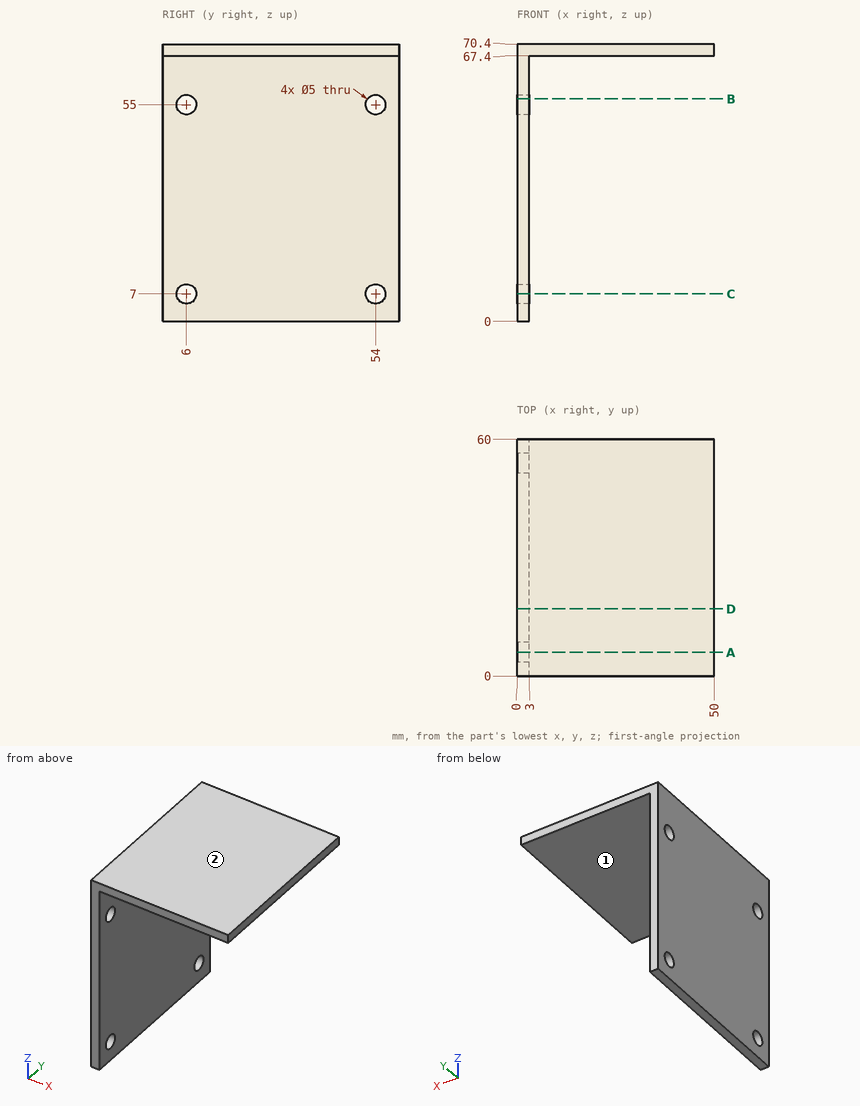
Job drawing, mm, ordinate dimensions from the low corner. One solid piece. A direction names the side the tool comes from. Round coordinates to 2 decimals unless told otherwise and drop trailing zeros. Write each loop counter-clockwise with the first axis right and the second up, starting at its lowest first coordinate (ties: lowest second). Pieces come first, ordered by that corner, then holes. Notation, with made-up numbers: (-21.75, 63.25) -> (-3.75, 63.25) arc R16 ccw to (-3.75, 88.25) -> close; hole circle Ø3 at (2, -22). An arc over 180 degrees is marked (long way). Answer as a JSON object with one key per item and string values.
(1) Which spindle directions (+Z, -Z, +X, -X, +Y, -Y) get a long thin tool onto all of the face, cutting with end or side? Do the marked faces 1 and 2. Say none if no direction does.
Reported:
{"face 1": "-Z, +X, +Y, -Y", "face 2": "+Z, +X, -X, +Y, -Y"}
(2) Band-saw the part on D-D, the plane y = 17. List the corners of the cut face in (x, z), then the cut area to 3 significant figures.
Reported:
{"outline": "(0, 0) -> (3, 0) -> (3, 67.4) -> (50, 67.4) -> (50, 70.4) -> (0, 70.4) -> close", "area": "352 mm^2"}
(3) Probe probe 1 along Y at (x, z) = (1.65, 7); probe 2 along X at (y, z) = (54.5, 47); probe 3 along Z at (x, y) = (46, 7). List the from-to ranges inside material, lowest first. Write a range as [from, to].
Reported:
{"probe 1": "y = [0, 3.5], [8.5, 51.5], [56.5, 60]", "probe 2": "x = [0, 3]", "probe 3": "z = [67.4, 70.4]"}
(4) Band-saw the part on C-C, the plane z = 7. List the corners of the cut face in (x, y).
Reported:
{"outline": "(0, 0) -> (3, 0) -> (3, 3.5) -> (0, 3.5) -> close; (0, 8.5) -> (3, 8.5) -> (3, 51.5) -> (0, 51.5) -> close; (0, 56.5) -> (3, 56.5) -> (3, 60) -> (0, 60) -> close"}
(5) Pin check, flat tips, straight feed: P1, Ø14, axis at x = 20.5, y = 32, coming from the -Z side; P2, Ø6.5, axis at y = 54, z = 55, coming from the +X side. Stop position of each tip, or through.
Reported:
{"P1": "stops at z = 67.4", "P2": "stops at x = 3"}
(6) Band-saw the part on B-B, the plane z = 56.5. List the corners of the cut face in (x, y).
Reported:
{"outline": "(0, 0) -> (3, 0) -> (3, 4) -> (0, 4) -> close; (0, 8) -> (3, 8) -> (3, 52) -> (0, 52) -> close; (0, 56) -> (3, 56) -> (3, 60) -> (0, 60) -> close"}
(7) Band-saw the part on A-A, the plane y = 6. List the corners of the cut face in (x, z).
Reported:
{"outline": "(0, 0) -> (3, 0) -> (3, 4.5) -> (0, 4.5) -> close; (0, 9.5) -> (3, 9.5) -> (3, 52.5) -> (0, 52.5) -> close; (0, 57.5) -> (3, 57.5) -> (3, 67.4) -> (50, 67.4) -> (50, 70.4) -> (0, 70.4) -> close"}
